Autodesk Inventor part; units mm, degrees
ref_plane "Work Plane1" through (3, 0, 0) normal (1, 0, 0) x (0, 0, -1)
ref_plane "Work Plane2" through (0, 3, 0) normal (0, -1, 0) x (1, 0, 0)
ref_plane "YZ Plane" through (0, 0, 0) normal (1, 0, 0) x (0, 1, 0)
sketch "Sketch1" plane through (0, 0, 0) normal (0, 0, 1) x (1, 0, 0)
  line L0 (0, 0) -> (6, 0)
  line L1 (6, 0) -> (6, 6)
  line L2 (6, 6) -> (0, 6)
  line L3 (0, 6) -> (0, 0)
  dimension "d0" = 6
  dimension "d1" = 6
extrude "Extrusion1" add sketch "Sketch1" along normal blind 3.16
sketch "Sketch2" plane through (0, 0, 3.16) normal (0, 0, 1) x (1, 0, 0)
  circle A0 centre (3, 3) radius 1.735
  line L0 (6, 0) -> (6, 6)
  line L1 (6, 6) -> (0, 6)
  point P0 (0, 0)
  point P1 (6, 3)
  point P2 (3, 6)
  dimension "d4" = 3.47
extrude "Extrusion2" add sketch "Sketch2" along normal blind 1.84
sketch "Sketch3" plane through (0, 0, 0) normal (0, 0, -1) x (-1, 0, 0)
  line L0 (-5.6, 6.31) -> (-4.88, 6.31)
  line L1 (-4.88, 6.31) -> (-4.88, 6)
  line L2 (-4.88, 6) -> (-5.6, 6)
  line L3 (-5.6, 6) -> (-5.6, 6.31)
  line L4 (-6, 6) -> (0, 6)
  line L5 (-6, 0) -> (-6, 6)
  point P0 (0, 0)
  dimension "d7" = 0.72
  dimension "d8" = 0.31
  dimension "d9" = 0.4
extrude "Extrusion3" add sketch "Sketch3" along normal blind 3 and the other way blind 1
ref_plane "Work Plane1" through (3, 0, 0) normal (1, 0, 0) x (0, 0, -1)
ref_plane "Work Plane2" through (0, 3, 0) normal (0, -1, 0) x (1, 0, 0)
mirror "Mirror3" about plane through (3, 0, 0) normal (1, 0, 0) of "Extrusion3"
mirror "Mirror4" about plane through (0, 3, 0) normal (0, -1, 0) of "Extrusion3", "Mirror3"
properties part number "Button"
Part model, mm, in its own coordinate system. A direction names the side the tool comes from. Round coordinates to 2 decimals unless told otherwise and drop trailing zeros. Loops run counter-clockwise (first coordinate to the right, second up) from the corner with the lowest first, then second, coordinate; pieces in that order, holes last.
1. Two-plate mould, pull along Y, no slides. Class faces 3 (the face through (3, 3, 5)), 4 (the face through (4.655, 2.479, 4.067)), 5 (the face through (3, 3, 0)): pulls with the +Y half, pulls with the -Y half, needs draft (parallel to the pull), parting line crosses it, or undercut.
Solutions:
face 3: needs draft
face 4: parting line crosses it
face 5: undercut
2. 3-axis set-ups, long thin cutter, end or side, ignore diameter. For faces 1 (the face through (0, 3, 2)), 2 (the face through (1.6, 4.4, 3.16)): which of +Z, -Z, +X, -X, +Y, -Y reach the whole face in a straight line?
Solutions:
face 1: +Z, -Z, -X, +Y, -Y
face 2: +Z
3. Slice it at B-B (y = 3). Give the cut face in (x, z) (3 decimals), and give its area (3 significant figures).
Solutions:
outline: (0, 0) - (6, 0) - (6, 3.16) - (4.735, 3.16) - (4.735, 5) - (1.265, 5) - (1.265, 3.16) - (0, 3.16) - close
area: 25.3 mm2
4. Flat gauge pins, fed straight in: pin 1 (1 mm diameter, centred on x = 3.5, z = -2, fed in from +Y); pin 2 (3 mm diameter, centred on x = 3, y = 1.5, fed in from -Z); pin 3 (1.5 mm diameter, centred on x = 2, z = 4, fed in from +Y). Where does each tip first touch, or does it go through?
Solutions:
pin 1: passes through
pin 2: stops at z = 0
pin 3: stops at y = 4.72
5. Slice it at A-A (z = 0.25). Give the cut face in (x, y).
Solutions:
outline: (0, 0) - (0.4, 0) - (0.4, -0.31) - (1.12, -0.31) - (1.12, 0) - (4.88, 0) - (4.88, -0.31) - (5.6, -0.31) - (5.6, 0) - (6, 0) - (6, 6) - (5.6, 6) - (5.6, 6.31) - (4.88, 6.31) - (4.88, 6) - (1.12, 6) - (1.12, 6.31) - (0.4, 6.31) - (0.4, 6) - (0, 6) - close
6. Drill centre lines: line 1 along Y through (x, z) = (5.55, -0.25); line 2 along Z through (x, y) = (3.35, 4.25); line 3 along Z through (x, y) = (3.4, 0.5). Where is each one in solid material? Low to high.
Solutions:
line 1: y = -0.31 to 0, 6 to 6.31
line 2: z = 0 to 5
line 3: z = 0 to 3.16
7. Slice it at D-D (x = 5.05). Give the cut face in (y, z).
Solutions:
outline: (-0.31, -3) - (0, -3) - (0, 0) - (6, 0) - (6, -3) - (6.31, -3) - (6.31, 1) - (6, 1) - (6, 3.16) - (0, 3.16) - (0, 1) - (-0.31, 1) - close
